Read the model definition and answer for the solid it produces. Units are mm, in the model's axes. Give positions to 0.01 mm unless a question says otherwise; leave off trailing zeros. Order: outer loops, then holes, each group sorted by start corner. A loop starts at its lowest first (then second) coordinate and runs counter-clockwise, first axis right, second up. Notation, with made-up numbers: M 83,-29 L 95,-29 A17 ccw 95,-25 Z; hole C 79.25,11.5 d8. An arc over 180 degrees is marked long. One line per item, written item: value.
from build123d import *

# Parameters (mm, degrees)
F2_R      = 3.96875
F3_DEPTH  = 19.05
F3_FACE_R = 3.96875
F5_R      = 3.96875
F6_DEPTH  = 9.525
F7_R      = 3.96875
F8_DEPTH  = 3.175
F8_TAPER  = 60


# Not quite as in the source:
# - an extrude whose draft closes it to a point is written as a loft to that point


with BuildPart() as f1:
    # F0 (on Front) → F1 (revolve)
    with BuildSketch(Plane.XZ):
        with BuildLine():
            Line((0, 0), (12.7, 0))
            ThreePointArc((12.7, 0), (14.1990316571, 16.6245158286), (0, 25.4))
            Line((0, 25.4), (0, 0))
        make_face()
    revolve(axis=Axis((0, 0, 12.7), (0, 0, 1)))

    # F2 (on face) → F3 (cut)
    with BuildSketch(Plane(origin=(0, 0, 0), x_dir=(1, 0, 0), z_dir=(0, 0, -1))):
        Circle(F2_R)
    extrude(amount=-F3_DEPTH, mode=Mode.SUBTRACT)

    # F3_face (on face) → F4 section 0
    with BuildSketch(Plane(origin=(0, 0, 19.05), x_dir=(1, 0, 0), z_dir=(0, 0, -1)), mode=Mode.PRIVATE) as f4_s0:
        Circle(F3_FACE_R)
    loft([f4_s0.sketch, Vertex(0, 0, 23.01875)], ruled=True, mode=Mode.SUBTRACT)

    # F5 (on face) → F6 (cut)
    with BuildSketch(Plane(origin=(0, 0, 0), x_dir=(1, 0, 0), z_dir=(0, 0, -1))):
        Polygon((-8.5, 4.9074772881), (-8.5, -4.9074772881), (0, -9.8149545762), (8.5, -4.9074772881), (8.5, 4.9074772881), (0, 9.8149545762), align=None)
        Circle(F5_R, mode=Mode.SUBTRACT)
    extrude(amount=-F6_DEPTH, mode=Mode.SUBTRACT)

    # F7 (on face) → F8 (cut)
    with BuildSketch(Plane(origin=(0, 0, 9.525), x_dir=(1, 0, 0), z_dir=(0, 0, -1))):
        Polygon((8.5, 4.9074772881), (0, 9.8149545762), (-8.5, 4.9074772881), (-8.5, -4.9074772881), (0, -9.8149545762), (8.5, -4.9074772881), align=None)
        Circle(F7_R, mode=Mode.SUBTRACT)
        Circle(F7_R)
    extrude(amount=-F8_DEPTH, taper=F8_TAPER, mode=Mode.SUBTRACT)


solid = f1.part
1) Find section C-C, the plane z = 14.75. Write down the section's boundary in (x, y), plus the area to 3 significant figures.
Reported:
outline: C 0,0 d29.98; hole C 0,0 d7.94
area: 656 mm^2
2) Each of these flat-tipped pins is pushed along its axis until it touches: pin 1 Ø1.5 at (y, z) = (-5, 8.5) entering from -X; pin 2 Ø1.5 at (y, z) = (8, 22.5) entering from +X; pin 3 Ø12 at (y, z) = (-8, 20) entering from -X. Where does it stop, or does it pass through?
Reported:
pin 1: stops at x = -15.27
pin 2: stops at x = 6.48
pin 3: stops at x = -14.16
3) Find section A-A, the plane z = 3.5. Write down the section's boundary in (x, y).
Reported:
outline: C 0,0 d29.37; hole M -8.5,-4.91 L 0,-9.81 L 8.5,-4.91 L 8.5,4.91 L 0,9.81 L -8.5,4.91 Z
4) Find section B-B, the plane y = -10.5. Write down the section's boundary in (x, z) (3 decimals).
Reported:
outline: M -7.144,0 L 7.144,0 A11.907 ccw long Z
5) Consider probe 1 along Y at (x, z) = (-1.5, 17); probe 2 along Y at (x, z) = (0, 15.75); probe 3 along X at (y, z) = (0, 16.25). Determine where each line is inside the solid, lowest interval first.
Reported:
probe 1: y = -13.92 to -3.67, 3.67 to 13.92
probe 2: y = -14.6 to -3.97, 3.97 to 14.6
probe 3: x = -14.38 to -3.97, 3.97 to 14.38
6) Determine the mould class of faces 1 (the face through (3, -8.3, 0)), 2 (the face through (4.31, -7.327, 4.696)), 3 (the face through (-4.31, 7.327, 4.696)) for opening direction X: +X half, -X half, draft (parallel to the pull), parting line (faces both ways), or undercut.
Reported:
face 1: draft
face 2: undercut
face 3: undercut
7) Find section D-D, the plane z = 17.75. Write down the section's boundary in (x, y), plus the area to 3 significant figures.
Reported:
outline: C 0,0 d27.16; hole C 0,0 d7.94
area: 530 mm^2
